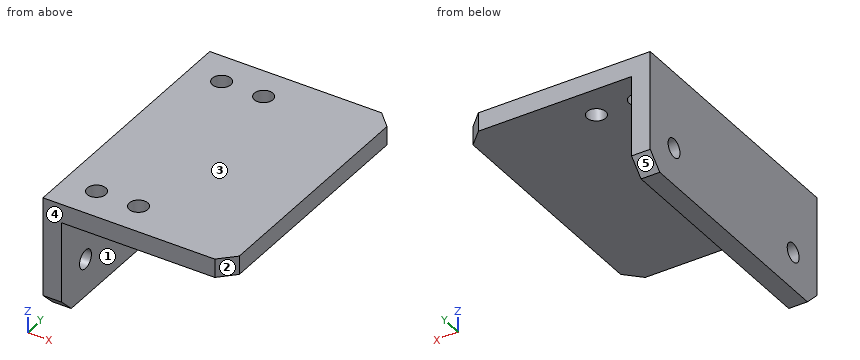
from build123d import *

# Parameters (mm, degrees)
F1_DEPTH = 88.9
F3_D     = 6.35
F4_SIZE  = 5.08
F6_D     = 6.35


with BuildPart() as f1:
    # F0 (on Front) → F1 (new body)
    with BuildSketch(Plane.XZ):
        Polygon((0, 38.8874), (0, 0), (6.35, 0), (6.35, 32.5374), (63.5, 32.5374), (63.5, 38.8874), align=None)
    extrude(amount=F1_DEPTH)

    # F3 (through all)
    with Locations(Plane.YZ.offset(6.35)):
        with Locations((-76.2, 12.7), (-12.7, 12.7)):
            Hole(F3_D / 2)

    # F4
    f4_edges = [f1.edges().sort_by_distance(p)[0] for p in [
        (3.175, -88.9, 0),
        (63.5, -88.9, 35.7124),
        (63.5, 0, 35.7124),
        (3.175, 0, 0),
    ]]
    chamfer(f4_edges, length=F4_SIZE)

    # F6 (through all)
    with Locations(Plane.XY.offset(38.8874)):
        with Locations((25.4, -11.1252), (11.1252, -11.1252), (11.1252, -77.8002), (25.4, -77.8002)):
            Hole(F6_D / 2)


solid = f1.part
CAD build for the part. Positions are in the model's coordinates, mm. Face numbers are marked on the shaded views. A direction names the side the tool comes from. Coordinates: 2 decimals unless noted, no trailing zeros. Write each loop counter-clockwise with the first axis right and the second up, starting at its lowest first coordinate (ties: lowest second). Pieces come first, ordered by that corner, then holes. Notation, with made-up numbers: M 78.25,6.5 L 98.25,6.5 A34 ccw 98.25,40.5 Z; hole C 27.5,-20.5 d8. An arc over 180 degrees is marked long. Answer as a JSON object with one key per item and string values. Group by question number.
1) Saw through at D-D (z = 22). Write the cut outline in (x, y), plus the area to 3 significant figures.
2) Saw through at C-C (y = -12.7). Write the cut outline in (x, z) (3 decimals).
3) Saw through at A-A (z = 12.7). Write the cut outline in (x, y) (3 decimals).
4) Pin check, flat tips, straight feed: pin 1 Ø8.5 at (y, z) = (-12.7, 12.7) entering from +X; pin 2 Ø4 at (x, y) = (40, -32.5) entering from -Z; pin 3 Ø10 at (x, y) = (11.13, -77.8) entering from -Z. Stop position of each tip, or through.
5) Wall check: line 1 (Y direction, x = 25.4, z = 35); line 2 (Z direction, x = 5, y = -76.2) (3 decimals); line 3 (Z direction, x = 21, y = -70). Give the ranges that are in metal, low to high. Write a range as from..to.
6) Saw through at B-B (x = 5). Write the cut outline in (y, z) (3 decimals).
7) Tool access for the marked faces 1 and 2: list every direction of +Z, -Z, +X, -X, +Y, -Y with a clear straight run to the whole face (end or side of a thin tool).
8) Mould opens along Y. For the marked faces 3, 4 and 5 say: +Y half, -Y half, draft (parallel to the pull), parting line (faces both ways), or undercut.
Values follow:
{
 "1": {"outline": "M 0,-88.9 L 6.35,-88.9 L 6.35,0 L 0,0 Z", "area": "565 mm2"},
 "2": {"outline": "M 0,0 L 6.35,0 L 6.35,9.525 L 0,9.525 Z; M 0,15.875 L 6.35,15.875 L 6.35,32.537 L 8.368,32.537 L 8.368,38.887 L 0,38.887 Z; M 13.882,32.537 L 22.643,32.537 L 22.643,38.887 L 13.882,38.887 Z; M 28.157,32.537 L 63.5,32.537 L 63.5,38.887 L 28.157,38.887 Z"},
 "3": {"outline": "M 0,-88.9 L 6.35,-88.9 L 6.35,-79.375 L 0,-79.375 Z; M 0,-73.025 L 6.35,-73.025 L 6.35,-15.875 L 0,-15.875 Z; M 0,-9.525 L 6.35,-9.525 L 6.35,0 L 0,0 Z"},
 "4": {"pin 1": "stops at x = 6.35", "pin 2": "stops at z = 32.54", "pin 3": "stops at z = 0"},
 "5": {"line 1": "y = -88.9..-80.98, -74.63..-14.3, -7.95..0", "line 2": "z = 0..9.525, 15.875..38.887", "line 3": "z = 32.54..38.89"},
 "6": {"outline": "M -88.9,5.08 L -83.82,0 L -5.08,0 L 0,5.08 L 0,38.887 L -88.9,38.887 Z; hole C -76.2,12.7 d6.35; hole C -12.7,12.7 d6.35"},
 "7": {"face 1": "-Z, +X, +Y, -Y", "face 2": "+Z, -Z, +X, -Y"},
 "8": {"face 3": "draft", "face 4": "-Y half", "face 5": "+Y half"}
}
